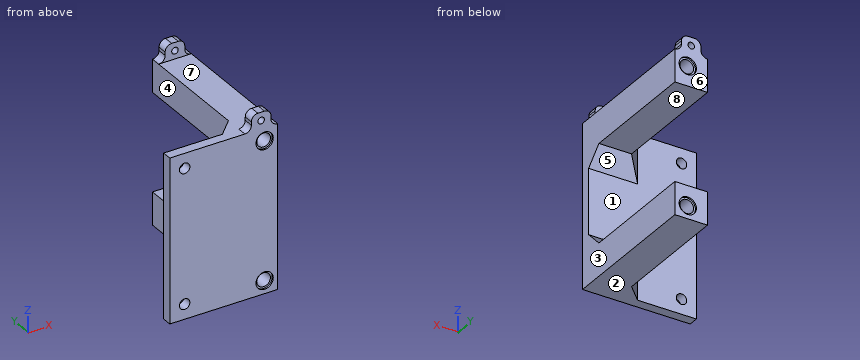
from build123d import *

# Parameters (mm, degrees)
SKETCH1_R           = 1.6
BOSS_EXTRUDE1_DEPTH = 3
SKETCH2_W           = 10
SKETCH2_H           = 10
BOSS_EXTRUDE2_DEPTH = 42
CHAMFER1_SIZE       = 5
SKETCH3_R           = 2.1
CUT_EXTRUDE1_DEPTH  = 52
SKETCH4_R           = 2.65
CUT_EXTRUDE2_DEPTH  = 0.5
SKETCH11_W          = 6
SKETCH11_H          = 3
BOSS_EXTRUDE7_DEPTH = 5
SKETCH12_R          = 1
CUT_EXTRUDE5_DEPTH  = 70.137227445
FILLET1_R           = 2


with BuildPart() as part:
    # Sketch1 → Boss-Extrude1 (new body)
    with BuildSketch(Plane(origin=(0, 0, 0), x_dir=(1, 0, 0), z_dir=(0, 1, 0))):
        Polygon((-6.512396694, 9.685950413), (1.487603306, 9.685950413), (26.487603306, 9.685950413), (26.487603306, -40.314049587), (1.487603306, -40.314049587), (-6.512396694, -40.314049587), align=None)
        with Locations(Location((-1.962396694, -35.764049587, 0), (0, 0, 270))):
            Circle(SKETCH1_R, mode=Mode.SUBTRACT)
        with Locations(Location((-1.962396694, 5.135950413, 0), (0, 0, 270))):
            Circle(SKETCH1_R, mode=Mode.SUBTRACT)
    extrude(amount=BOSS_EXTRUDE1_DEPTH)

    # Sketch2 → Boss-Extrude2 (add)
    with BuildSketch(Plane(origin=(0, 3, 0), x_dir=(1, 0, 0), z_dir=(0, 1, 0))):
        with Locations((21.487603306, -35.314049587)):
            Rectangle(SKETCH2_W, SKETCH2_H)
        with Locations((21.487603306, 4.685950413)):
            Rectangle(SKETCH2_W, SKETCH2_H)
    extrude(amount=BOSS_EXTRUDE2_DEPTH)

    # Chamfer1
    chamfer1_edges = [part.edges().sort_by_distance(p)[0] for p in [
        (21.487603306, 3, 30.314049587),
        (16.487603306, 3, 35.314049587),
        (16.487603306, 3, -4.685950413),
        (21.487603306, 3, 0.314049587),
    ]]
    chamfer(chamfer1_edges, length=CHAMFER1_SIZE)

    # Sketch3 → Cut-Extrude1 (cut)
    with BuildSketch(Plane(origin=(0, 45, 0), x_dir=(1, 0, 0), z_dir=(0, 1, 0))):
        with Locations(Location((22.537603306, -36.364049587, 0), (0, 0, 270))):
            Circle(SKETCH3_R)
        with Locations(Location((22.537603306, 5.735950413, 0), (0, 0, 270))):
            Circle(SKETCH3_R)
    extrude(amount=-CUT_EXTRUDE1_DEPTH, mode=Mode.SUBTRACT)

    # Sketch4 → Cut-Extrude2 (cut)
    with BuildSketch(Plane(origin=(0, 45, 0), x_dir=(1, 0, 0), z_dir=(0, 1, 0))):
        with Locations(Location((22.537603306, -36.364049587, 0), (0, 0, 270))):
            Circle(SKETCH4_R)
        with Locations(Location((22.537603306, 5.735950413, 0), (0, 0, 270))):
            Circle(SKETCH4_R)
    cut_extrude2 = extrude(amount=-CUT_EXTRUDE2_DEPTH, mode=Mode.SUBTRACT)

    # Mirror1: Cut-Extrude2 across plane
    add(cut_extrude2.mirror(Plane(origin=(0, 22.5, 0), x_dir=(0, 0, 1), z_dir=(0, -1, 0))), mode=Mode.SUBTRACT)

    # Sketch11 → Boss-Extrude7 (add)
    with BuildSketch(Plane.XY.offset(40.314049587)):
        with Locations((21.487603306, 43.5)):
            Rectangle(SKETCH11_W, SKETCH11_H)
        with Locations((21.487603306, 1.5)):
            Rectangle(SKETCH11_W, SKETCH11_H)
    extrude(amount=BOSS_EXTRUDE7_DEPTH)

    # Sketch12 → Cut-Extrude5 (cut, through all)
    with BuildSketch(Plane.XZ):
        with Locations(Location((21.487603306, 42.814049587, 0), (0, 0, 270))):
            Circle(SKETCH12_R)
    extrude(amount=-CUT_EXTRUDE5_DEPTH, mode=Mode.SUBTRACT)

    # Fillet1
    fillet1_edges = [part.edges().sort_by_distance(p)[0] for p in [
        (18.487603306, 43.5, 40.314049587),
        (24.487603306, 43.5, 40.314049587),
        (18.487603306, 1.5, 40.314049587),
        (24.487603306, 1.5, 40.314049587),
    ]]
    fillet(fillet1_edges, radius=FILLET1_R - 0.0001)  # a hair under: the kernel refuses the full size
    fillet1_2_edges = [part.edges().sort_by_distance(p)[0] for p in [
        (18.487603306, 43.5, 45.314049587),
        (24.487603306, 43.5, 45.314049587),
        (24.487603306, 1.5, 45.314049587),
        (18.487603306, 1.5, 45.314049587),
    ]]
    fillet(fillet1_2_edges, radius=FILLET1_R)


solid = part.part
Source: CAD feature listing. Evaluate the final solid. Frame: model axes, mm. Face numbers are marked on the shaded views. A direction names the side the tool comes from. Give positions to 0.01 mm unless a question says otherwise; leave off trailing zeros. Write each loop counter-clockwise with the first axis right and the second up, starting at its lowest first coordinate (ties: lowest second). Pieces come first, ordered by that corner, then holes. Notation, with made-up numbers: M -22.5,2 L 22.5,2 A20 ccw 22.5,9 Z; hole C -25,-6 d9. An arc over 180 degrees is marked long. Answer as a JSON object with one key per item and string values.
Q1. Cut plane B-B, the plane x = 12.5. Return the cut outline in (y, z).
Geometry check:
{"outline": "M 0,-9.69 L 4.01,-9.69 L 4.01,4.3 L 3,5.31 L 3,25.31 L 4.01,26.33 L 4.01,40.31 L 0,40.31 Z"}
Q2. Ray query, line 1 along Z through (x, y) = (23, 11); line 2 along Y through (x, z) = (17, 23); line 3 along X through (y, z) = (12, 33). Return the intervals inside material, ascending.
Geometry check:
{"line 1": "z = -9.69 to -7.78, -3.69 to 0.31, 30.31 to 34.32, 38.41 to 40.31", "line 2": "y = 0 to 3", "line 3": "x = 16.49 to 26.49"}
Q3. Access query for the marked faces 1, 2, 3, 4 and 5. Directions: +Z, -Z, +X, -X, +Y, -Y. A direction counts if a zero-diameter tool reaches every point of the face in a straight line with its end or side. Return the directions, or none.
Geometry check:
{"face 1": "-X, +Y", "face 2": "-Z, +X, -X, +Y, -Y", "face 3": "+Z, -Z, +X, +Y, -Y", "face 4": "+Z, -Z, -X, +Y", "face 5": "+X, -X, +Y"}
Q4. Cut plane D-D, the plane x = 0.5. Return the cut outline in (y, z).
Geometry check:
{"outline": "M 0,-9.69 L 3,-9.69 L 3,40.31 L 0,40.31 Z"}
Q5. Cut plane C-C, the plane z = 11. Return the cut outline in (x, y), then the cut area to 3 significant figures.
Geometry check:
{"outline": "M -6.51,0 L 26.49,0 L 26.49,3 L -6.51,3 Z", "area": "99.0 mm^2"}
Q6. Contact query for flat-ended pins moving along their axis: P1, Ø3, axis at x = 3, z = 37, coming from the +Y side; P2, Ø4, axis at x = 22.54, z = 36.36, coming from the +Y side; P3, Ø6, axis at x = 15, y = 31, coming from the +Z side; P4, Ø6, axis at x = 22.54, z = -5.74, coming from the +Y side. Output: stop coordinate, or through.
Geometry check:
{"P1": "stops at y = 3", "P2": "passes through", "P3": "stops at z = 40.31", "P4": "stops at y = 45"}
Q7. Mould query, pull axis Y, two halves, no side actions, for the marked faces 6, 7 and 8. Classes: +Y half, -Y half, draft (parallel to the pull), parting line (faces both ways), or undercut.
Geometry check:
{"face 6": "+Y half", "face 7": "undercut", "face 8": "draft"}
Q8. Cut plane A-A, the plane y = 39. Return the cut outline in (x, z).
Geometry check:
{"outline": "M 16.49,-9.69 L 26.49,-9.69 L 26.49,0.31 L 16.49,0.31 Z; M 16.49,30.31 L 26.49,30.31 L 26.49,40.31 L 16.49,40.31 Z; hole C 22.54,-5.74 d4.2; hole C 22.54,36.36 d4.2"}
